Geometry check sheet. Reference: drawing and pictorial views, mm from the part's lowest x, y, z. A direction names the side the tool comes from. Round coordinates to 2 decimals unless told otherwise and drop trailing zeros. Order: outer loops, then holes, each group sorted by start corner. A loop starts at its lowest first (then second) coordinate and runs counter-clockwise, first axis right, second up.
Q1. Cross-section at D-D on y = 42. Record the cut outline in (x, z).
Q2. Scan lines: probe 1 along Z at (x, y) = (13, 18); probe 2 along X at (y, z) = (10, 2.5) (1 decimal); probe 3 along X at (y, z) = (24, 2.5) (1 decimal). Record each from-to range of solid material in increasing order.
Q3. Mould release check, pull along X, two halves, no side actions. Record for the marked faces 3, 4 and 5: +X half, -X half, draft (parallel to the pull), parting line (faces both ways), or undercut.
Q4. Set-up check for the marked faces 1 and 2: record each of +Z, -Z, +X, -X, +Y, -Y from which the full face is reachable in a straight line by a thin tool's end or side.
Q5. Depth check by flat-ended pin: P1, Ø13.5, axis at x = 28, y = 21.5, coming from the +Z side; P2, Ø1.6, axis at x = 23, z = 1, coming from the -Y side; P3, Ø2, axis at x = 23.5, z = 1, coming from the +Y side. Enter the tip coordinate at first touch or a pass-through.
Q6. Cross-section at C-C on z = 4. Record the cut outline in (x, y) (1 decimal).
Q7. Cross-section at A-A on y = 33. Record the cut outline in (x, z).
Q8. Cross-section at B-B on x = 21. Record the cut outline in (y, z) (1 decimal).
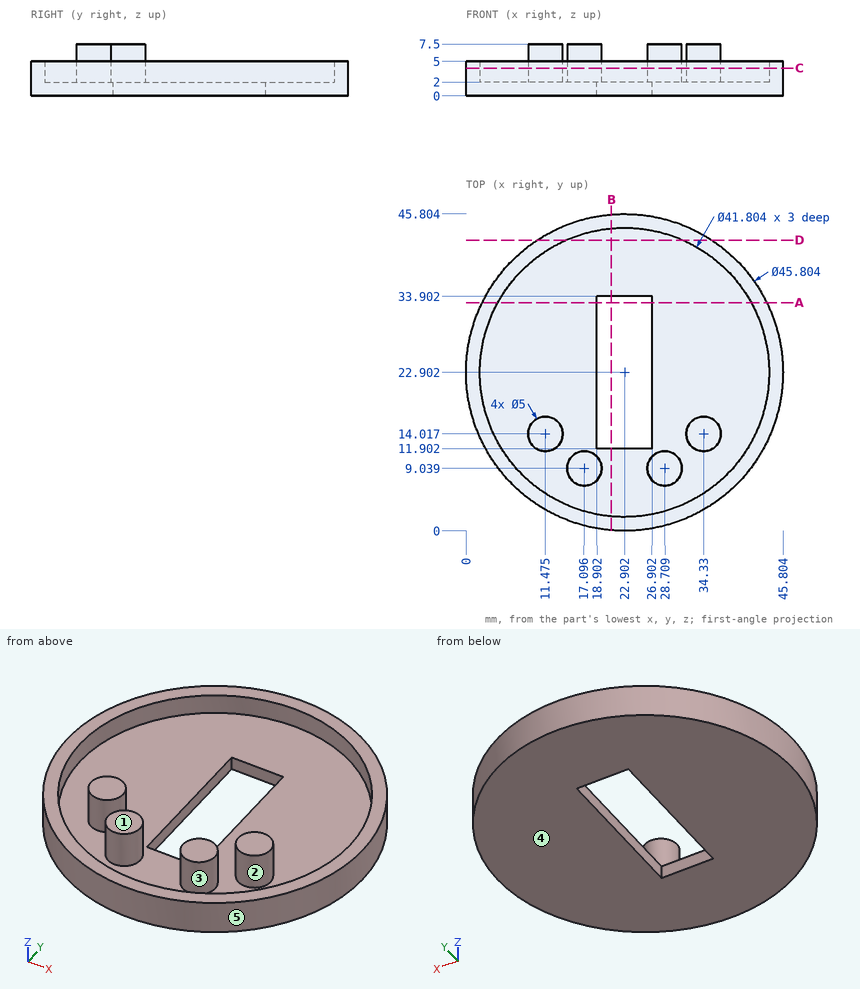
Results found:
1. outline: (10.26, 0) - (35.54, 0) - (35.54, 5) - (31.4, 5) - (31.4, 2) - (14.41, 2) - (14.41, 5) - (10.26, 5) - close
2. probe 1: z = 0 to 2
2. probe 2: x = 4 to 6.5, 14.8 to 19.4, 26.4 to 31, 39.3 to 41.8
2. probe 3: x = 0 to 2, 43.8 to 45.8
3. face 3: undercut
3. face 4: draft
3. face 5: parting line
4. face 1: +Z, +X, -X, +Y, -Y
4. face 2: +Z
5. P1: stops at z = 2
5. P2: stops at y = 0
5. P3: stops at y = 45.8
6. outline: circle Ø45.8 at (22.9, 22.9); circle Ø5 at (11.5, 14); circle Ø5 at (17.1, 9); circle Ø5 at (28.7, 9); circle Ø5 at (34.3, 14); hole circle Ø41.8 at (22.9, 22.9)
7. outline: (2.35, 0) - (18.9, 0) - (18.9, 2) - (4.6, 2) - (4.6, 5) - (2.35, 5) - close; (26.9, 0) - (43.46, 0) - (43.46, 5) - (41.2, 5) - (41.2, 2) - (26.9, 2) - close
8. outline: (0.1, 0) - (11.9, 0) - (11.9, 2) - (2.1, 2) - (2.1, 5) - (0.1, 5) - close; (33.9, 0) - (45.7, 0) - (45.7, 5) - (43.7, 5) - (43.7, 2) - (33.9, 2) - close
